Part model, mm, in its own coordinate system. A direction names the side the tool comes from. Coordinates: 2 decimals unless noted, no trailing zeros. Loops run counter-clockwise (first coordinate to the right, second up) from the corner with the lowest first, then second, coordinate; pieces in that order, holes last. Notation, with made-up numbers: M 58,36.5 L 112,36.5 A11 cw 112,55.5 Z; hole C -29.5,-12 d10. An arc over 180 degrees is marked long. Answer as a JSON object with one key per item and string values. Group by question number.
1. 3-axis set-ups, long thin cutter, end or side, ignore diameter. For faces 4 (the face through (0.52, 47.157, -13.43)), 5 (the face through (7.564, 45.563, -6.413)), 6 (the face through (-7.564, 43.087, 2.008)): which of +Z, -Z, +X, -X, +Y, -Y reach the whole face in a straight line?
2. Saw through at D-D on z = 4. Write the cut outline in (x, y).
3. Drill centre lines: L1, parallel to Y at x = 0, z = -12.5; L2, parallel to X at y = 20.5, z = 0; L3, parallel to Y at x = 1.75, z = -17.5. Where is each one in solid material? Low to high.
4. Mould opens along Y. For faces 1 (the face through (-2.024, 20.213, -1.29)), 2 (the face through (0, 41, -8)), 3 (the face through (0, 50, -8.5)) say: released by +Y, released by -Y, zero draft, split by the parting line, or undercut.
5. Saw through at B-B on z = 0. Write the cut outline in (x, y), then the cut area to 3 significant figures.
6. Saw through at C-C on y = 7. Write the cut outline in (x, z).
7. Saw through at A-A on z = -16. Write the cut outline in (x, y).
8. Drop flat-ended pins along their axis: pin 1 Ø2 at (x, y) = (-3.5, 27.5) entering from -Z; pin 2 Ø2.5 at (x, y) = (0, 49.5) entering from -Z; pin 3 Ø2 at (y, z) = (39, -1.5) entering from -X. Give the stop position or say it passes through.
from build123d import *

# Parameters (mm, degrees)
SKETCH1_R           = 7.5
SKETCH1_R_2         = 2.4
BOSS_EXTRUDE1_DEPTH = 58
SKETCH2_W           = 17
SKETCH2_H           = 17
BOSS_EXTRUDE2_DEPTH = 17
SKETCH3_R           = 7.5
SKETCH3_R_2         = 2.4
BOSS_EXTRUDE3_DEPTH = 10
FILLET5_R           = 8
CHAMFER1_SIZE       = 10
FILLET4_R           = 5


with BuildPart() as part:
    # Sketch1 → Boss-Extrude1 (new body)
    with BuildSketch(Plane(origin=(0, 0, 0), x_dir=(1, 0, 0), z_dir=(0, 1, 0))):
        with Locations(Location((0, 0, 0), (0, 0, 90))):
            Circle(SKETCH1_R)
        with Locations(Location((0, 0, 0), (0, 0, 90))):
            Circle(SKETCH1_R_2, mode=Mode.SUBTRACT)
    extrude(amount=BOSS_EXTRUDE1_DEPTH)

    # Sketch2 → Boss-Extrude2 (add)
    with BuildSketch(Plane(origin=(0, 58, 0), x_dir=(1, 0, 0), z_dir=(0, 1, 0))):
        Rectangle(SKETCH2_W, SKETCH2_H)
    extrude(amount=-BOSS_EXTRUDE2_DEPTH)

    # Sketch3 → Boss-Extrude3 (add)
    with BuildSketch(Plane(origin=(0, 0, -8.5), x_dir=(-1, 0, 0), z_dir=(0, 0, -1))):
        with Locations((0, 49.5)):
            Circle(SKETCH3_R)
        with Locations((0, 49.5)):
            Circle(SKETCH3_R_2, mode=Mode.SUBTRACT)
    extrude(amount=BOSS_EXTRUDE3_DEPTH)

    # Fillet5
    fillet5_edges = [part.edges().sort_by_distance(p)[0] for p in [
        (8.5, 58, 0),
        (-8.5, 58, 0),
    ]]
    fillet(fillet5_edges, radius=FILLET5_R)

    # Chamfer1
    # the kernel refuses this chamfer: 10 mm, written as the material it takes off along each edge
    with BuildSketch(Plane(origin=(26.21682988, 58, 8.5), x_dir=(0, 0.027495876610586317, -0.9996219169112968), z_dir=(-1, 0, 0))) as chamfer1_piece_1:
        Polygon((CHAMFER1_SIZE * 0.999621916911, CHAMFER1_SIZE * 0.0274958766106), (-CHAMFER1_SIZE * 0.0274958766106, CHAMFER1_SIZE * 0.999621916911), (0, 0), align=None)
    extrude(amount=52.433659759, mode=Mode.SUBTRACT)

    # Fillet4
    # the kernel refuses this fillet: 5 mm, written as the material it takes off along each edge
    with BuildSketch(Plane(origin=(-8.5, 50, -8.5), x_dir=(1, 0, 0), z_dir=(0, -1, 0))) as fillet4_piece_1_section:
        with BuildLine():
            CenterArc((FILLET4_R, FILLET4_R), FILLET4_R, 180, 90)
            Line((0, FILLET4_R), (0, 0))
            Line((0, 0), (FILLET4_R, 0))
        make_face()
    fillet4_piece_1 = extrude(amount=21.5, mode=Mode.PRIVATE)
    fillet4_piece_1 = fillet4_piece_1 - Plane(origin=(0, 49.5, -7.300599215), x_dir=(-1, 0, 0), z_dir=(0, 0, 1)) * Cylinder(7.5, 64, mode=Mode.PRIVATE)
    add(fillet4_piece_1, mode=Mode.SUBTRACT)
    with BuildSketch(Plane(origin=(8.5, 50, -8.5), x_dir=(-1, 0, 0), z_dir=(0, -1, 0))) as fillet4_piece_2_section:
        with BuildLine():
            CenterArc((FILLET4_R, -FILLET4_R), FILLET4_R, 90, 90)
            Line((0, -FILLET4_R), (0, 0))
            Line((0, 0), (FILLET4_R, 0))
        make_face()
    fillet4_piece_2 = extrude(amount=21.5, mode=Mode.PRIVATE)
    fillet4_piece_2 = fillet4_piece_2 - Plane(origin=(0, 49.5, -7.300599064), x_dir=(-1, 0, 0), z_dir=(0, 0, 1)) * Cylinder(7.5, 63, mode=Mode.PRIVATE)
    add(fillet4_piece_2, mode=Mode.SUBTRACT)
    with BuildSketch(Plane(origin=(8.5, 41, -21), x_dir=(-1, 0, 0), z_dir=(0, 0, 1))) as fillet4_piece_3_section:
        with BuildLine():
            CenterArc((FILLET4_R, -FILLET4_R), FILLET4_R, 90, 90)
            Line((0, -FILLET4_R), (0, 0))
            Line((0, 0), (FILLET4_R, 0))
        make_face()
    fillet4_piece_3 = extrude(amount=42, mode=Mode.PRIVATE)
    fillet4_piece_3 = fillet4_piece_3 - Plane(origin=(0, 41.109676193, 0), x_dir=(0, 0, -1), z_dir=(0, -1, 0)) * Cylinder(7.5, 104, mode=Mode.PRIVATE)
    add(fillet4_piece_3, mode=Mode.SUBTRACT)
    with BuildSketch(Plane(origin=(-8.5, 41, 21), x_dir=(0, 1, 0), z_dir=(0, 0, -1))) as fillet4_piece_4_section:
        with BuildLine():
            CenterArc((FILLET4_R, FILLET4_R), FILLET4_R, 180, 90)
            Line((0, FILLET4_R), (0, 0))
            Line((0, 0), (FILLET4_R, 0))
        make_face()
    fillet4_piece_4 = extrude(amount=42, mode=Mode.PRIVATE)
    fillet4_piece_4 = fillet4_piece_4 - Plane(origin=(0, 44.689641685, 0), x_dir=(0, 0, -1), z_dir=(0, -1, 0)) * Cylinder(7.5, 104, mode=Mode.PRIVATE)
    add(fillet4_piece_4, mode=Mode.SUBTRACT)
    with BuildSketch(Plane(origin=(0.5, 50, -8.5), x_dir=(1, 0, 0), z_dir=(0, -1, 0))) as fillet4_piece_5_section:
        with BuildLine():
            CenterArc((8 - FILLET4_R, FILLET4_R), FILLET4_R, 270, 90)
            Line((8, FILLET4_R), (8, 0))
            Line((8, 0), (8 - FILLET4_R, 0))
        make_face()
    fillet4_piece_5 = revolve(axis=Axis((0.5, 50, -8.5), (0, 0, 1)), revolution_arc=90, mode=Mode.PRIVATE)
    fillet4_piece_5 = fillet4_piece_5 - Plane(origin=(0, 49.5, -6.88973409), x_dir=(-1, 0, 0), z_dir=(0, 0, 1)) * Cylinder(7.5, 33, mode=Mode.PRIVATE)
    add(fillet4_piece_5, mode=Mode.SUBTRACT)
    with BuildSketch(Plane(origin=(-0.5, 58, -8.5), x_dir=(0, -1, 0), z_dir=(1, 0, 0))) as fillet4_piece_6_section:
        with BuildLine():
            CenterArc((FILLET4_R, -FILLET4_R), FILLET4_R, 90, 90)
            Line((0, -FILLET4_R), (0, 0))
            Line((0, 0), (FILLET4_R, 0))
        make_face()
    fillet4_piece_6 = extrude(amount=1, mode=Mode.PRIVATE)
    fillet4_piece_6 = fillet4_piece_6 - Plane(origin=(0, 49.5, -6.859352055), x_dir=(-1, 0, 0), z_dir=(0, 0, 1)) * Cylinder(7.5, 23, mode=Mode.PRIVATE)
    add(fillet4_piece_6, mode=Mode.SUBTRACT)
    with BuildSketch(Plane(origin=(-0.5, 50, -8.5), x_dir=(-1, 0, 0), z_dir=(0, -1, 0))) as fillet4_piece_7_section:
        with BuildLine():
            CenterArc((8 - FILLET4_R, -FILLET4_R), FILLET4_R, 0, 90)
            Line((8, -FILLET4_R), (8, 0))
            Line((8, 0), (8 - FILLET4_R, 0))
        make_face()
    fillet4_piece_7 = revolve(axis=Axis((-0.5, 50, -8.5), (0, 0, -1)), revolution_arc=90, mode=Mode.PRIVATE)
    fillet4_piece_7 = fillet4_piece_7 - Plane(origin=(0, 49.5, -6.889734089), x_dir=(-1, 0, 0), z_dir=(0, 0, 1)) * Cylinder(7.5, 32, mode=Mode.PRIVATE)
    add(fillet4_piece_7, mode=Mode.SUBTRACT)


solid = part.part
Outcome:
{
 "1": {"face 4": "-Z", "face 5": "-Z, +X, -Y", "face 6": "-X, -Y"},
 "2": {"outline": "M -8.5,46 A5 ccw -6.34,41.89 L -6.34,0 L 6.34,0 L 6.34,41.89 A5 ccw 8.5,46 L 8.5,50 A8 ccw 8.1,52.5 L -8.1,52.5 A8 ccw -8.5,50 Z"},
 "3": {"L1": "y = 42 to 47.1, 51.9 to 57", "L2": "x = -7.5 to -2.4, 2.4 to 7.5", "L3": "y = 42.21 to 47.86, 51.14 to 56.79"},
 "4": {"face 1": "zero draft", "face 2": "released by -Y", "face 3": "undercut"},
 "5": {"outline": "M -8.5,46 A5 ccw -7.5,43 L -7.5,0 L -2.4,0 L -2.4,41 L 2.4,41 L 2.4,0 L 7.5,0 L 7.5,43 A5 ccw 8.5,46 L 8.5,50 A8 ccw 5.16,56.5 L -5.16,56.5 A8 ccw -8.5,50 Z", "area": "663 mm²"},
 "6": {"outline": "C 0,0 d15; hole C 0,0 d4.8"},
 "7": {"outline": "C 0,49.5 d15; hole C 0,49.5 d4.8"},
 "8": {"pin 1": "stops at z = -7.07", "pin 2": "stops at z = -8.5", "pin 3": "stops at x = -7.48"}
}
